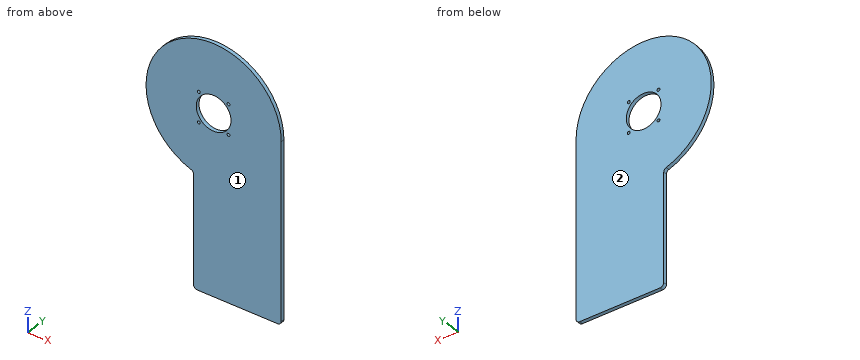
from build123d import *

# Parameters (mm, degrees)
F0_R     = 4
F0_R_2   = 47.5
F1_DEPTH = 10


with BuildPart() as f1:
    # F0 (on Front) → F1 (new body)
    with BuildSketch(Plane.XZ):
        with BuildLine():
            Line((370, 537.822554), (370, 1015))
            ThreePointArc((370, 1015), (78.1902, 1166.051867), (123.333333, 840.580327))
            ThreePointArc((123.333333, 840.580327), (128.164966, 836.92574), (130, 831.152237))
            Line((130, 831.152237), (130, 537.822554))
            ThreePointArc((130, 537.822554), (132.928932, 530.751486), (140, 527.822554))
            Line((140, 527.822554), (360, 527.822554))
            ThreePointArc((360, 527.822554), (367.071068, 530.751486), (370, 537.822554))
        make_face()
        with Locations((144.393782, 974.289006)):
            Circle(F0_R, mode=Mode.SUBTRACT)
        with Locations((144.289006, 1055.606218)):
            Circle(F0_R, mode=Mode.SUBTRACT)
        with Locations((225.710994, 974.393782)):
            Circle(F0_R, mode=Mode.SUBTRACT)
        with Locations((185, 1015)):
            Circle(F0_R_2, mode=Mode.SUBTRACT)
        with Locations((225.606218, 1055.710994)):
            Circle(F0_R, mode=Mode.SUBTRACT)
    extrude(amount=F1_DEPTH)


solid = f1.part
Design review of the part built by this model. Coordinates are the model's own, in mm. Face numbers are marked on the shaded views. Coordinates: 2 decimals unless noted, no trailing zeros. Loops run counter-clockwise (first coordinate to the right, second up) from the corner with the lowest first, then second, coordinate; pieces in that order, holes last.
Item 1: Draft analysis for pull direction Y (two halves, no side actions). For the marked faces 1 and 2, state which applies: pulls with the +Y half, pulls with the -Y half, needs draft (parallel to the pull), parting line crosses it, or undercut.
Completed:
face 1: pulls with the -Y half
face 2: pulls with the +Y half
Item 2: Add section B-B (y = -6.75). Write out the cut boundary in (x, z).
Completed:
outline: (123.33, 840.58) arc R10 cw to (130, 831.15) - (130, 537.82) arc R10 ccw to (140, 527.82) - (360, 527.82) arc R10 ccw to (370, 537.82) - (370, 1015) arc R185 ccw (long way) to start; hole circle Ø95 at (185, 1015); hole circle Ø8 at (144.29, 1055.61); hole circle Ø8 at (144.39, 974.29); hole circle Ø8 at (225.61, 1055.71); hole circle Ø8 at (225.71, 974.39)
Item 3: Add section A-A (x = 185). Write out the cut boundary in (y, z), and give its area (3 significant figures).
Completed:
outline: (-10, 527.82) - (0, 527.82) - (0, 967.5) - (-10, 967.5) - close; (-10, 1062.5) - (0, 1062.5) - (0, 1200) - (-10, 1200) - close
area: 5,770 mm2
Item 4: Add section D-D (x = 282). Write out the cut boundary in (y, z), and give its area (3 significant figures).
Completed:
outline: (-10, 527.82) - (0, 527.82) - (0, 1172.53) - (-10, 1172.53) - close
area: 6,450 mm2
Item 5: Wall thickness on L1, parallel to X at y = -2.75, z = 1015.5; L2, parallel to Z at x = 226.5, y = -0.5; L3, parallel to Z at x = 195, y = -6.5: over which ranges is each line inside the solid? List them lowest first.
Completed:
L1: x = 0 to 137.5, 232.5 to 370
L2: z = 527.82 to 970.47, 978.32 to 991.89, 1038.11 to 1051.81, 1059.61 to 1195.29
L3: z = 527.82 to 968.56, 1061.44 to 1199.73
Item 6: Clearance check with flat-ended pins moving along their axes: pin 1 (6 mm diameter, centred on y = -4, z = 799.5, fed in from -X); pin 2 (1.5 mm diameter, centred on x = 177, y = -5.5, fed in from +Z); pin 3 (6.5 mm diameter, centred on x = 144.39, z = 974.29, fed in from -Y). State where each tip first meets the part, or that it passes through.
Completed:
pin 1: stops at x = 130
pin 2: stops at z = 1199.86
pin 3: passes through
Item 7: Add section C-C (z = 581.5). Write out the cut boundary in (x, y), and give its area (3 significant figures).
Completed:
outline: (130, -10) - (370, -10) - (370, 0) - (130, 0) - close
area: 2,400 mm2
